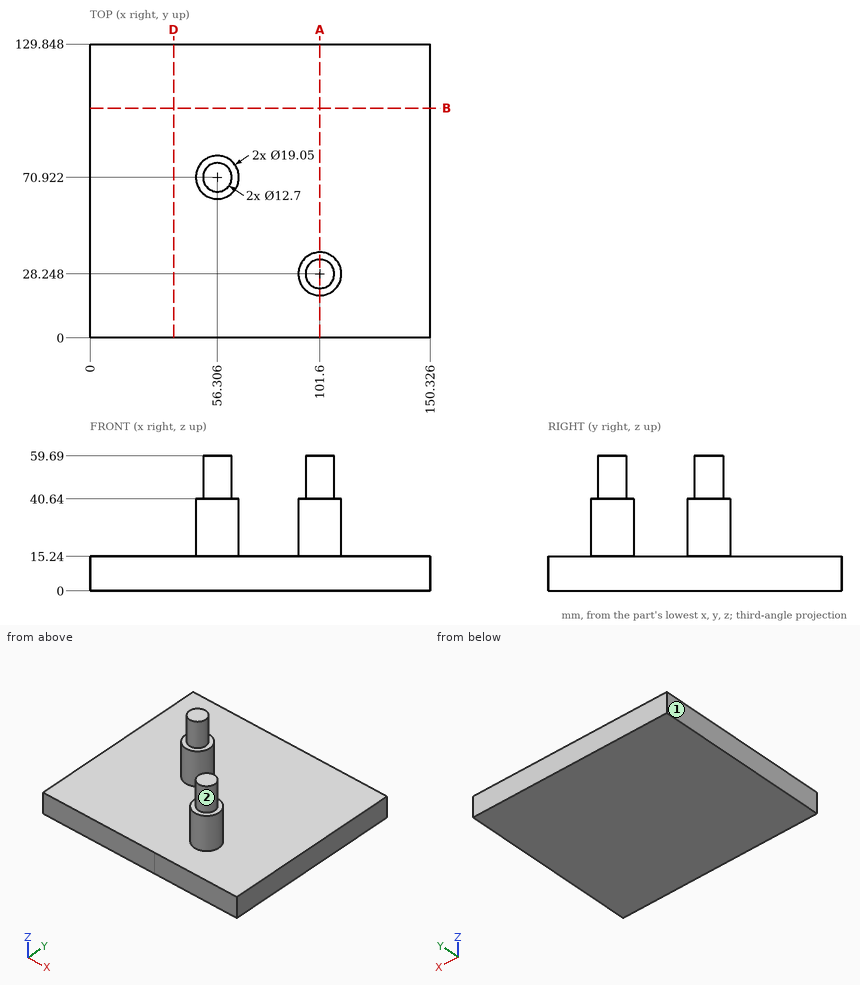
Geometry: see drawing. Coordinates: mm, zero at the bounding-box minimum. A direction names the side the tool comes from. Give positions to 0.01 mm unless a question says otherwise; leave off trailing zeros. Loops run counter-clockwise (first coordinate to the right, second up) from the corner with the lowest first, then second, coordinate; pieces in that order, holes last. Notation, with made-up numbers: (26.5, -2.75) -> (62.5, -2.75) arc R31 ccw to (62.5, 22.25) -> close; hole circle Ø9 at (70.25, 12). An arc over 180 degrees is marked (long way). Use CSV: the item, a comma, the result in double quotes.
(1) Cut plane B-B (y = 101.5). Output: boundary loops of the cut face in (x, z) (1 decimal), plus the area to 3 significant figures.
From the geometry:
outline,"(0, 0) -> (150.3, 0) -> (150.3, 15.2) -> (0, 15.2) -> close"
area,"2,290 mm^2"
(2) Ray query, line 1 along Z through (x, y) = (96.5, 42); line 2 along X through (y, z) = (64.5, 34); line 3 along Y through (x, z) = (104.5, 57). Return the intervals inside material, ascending. Write a range as [from, to].
From the geometry:
line 1,"[0, 15.24]"
line 2,"[49.27, 63.34]"
line 3,"[22.6, 33.9]"
(3) Access query for the marked faces 1 and 2. Directions: +Z, -Z, +X, -X, +Y, -Y. A direction counts if a zero-diameter tool reaches every point of the face in a straight line with its end or side. Return the directions, or none.
From the geometry:
face 1,"+Z, -Z, -X, +Y, -Y"
face 2,"+Z"
(4) Cut plane A-A (x = 101.6). Output: boundary loops of the cut face in (y, z).
From the geometry:
outline,"(0, 0) -> (129.85, 0) -> (129.85, 15.24) -> (37.77, 15.24) -> (37.77, 40.64) -> (34.6, 40.64) -> (34.6, 59.69) -> (21.9, 59.69) -> (21.9, 40.64) -> (18.72, 40.64) -> (18.72, 15.24) -> (0, 15.24) -> close"
(5) First-contact query: P1, Ø10, axis at x = 49, z = 45, coming from the -Y side; P2, Ø2, axis at x = 18, y = 39.5, coming from the +Z side; P3, Ø2, axis at y = 29, z = 42.5, coming from the -X side. Flat tips, straight axial feed; report the tip coordinate or a pass-through.
From the geometry:
P1,"y = 62.73"
P2,"z = 15.24"
P3,"x = 95.25"
(6) Cut plane D-D (x = 37). Output: boundary loops of the cut face in (y, z).
From the geometry:
outline,"(0, 0) -> (129.85, 0) -> (129.85, 15.24) -> (0, 15.24) -> close"
